Geometry: final body of the model. Coordinates: model frame, mm. A direction names the side the tool comes from. Coordinates: 2 decimals unless noted, no trailing zeros. Loops run counter-clockwise (first coordinate to the right, second up) from the corner with the lowest first, then second, coordinate; pieces in that order, holes last. Notation, with made-up numbers: (76.5, -35.5) - (111.5, -35.5) arc R13 cw to (111.5, -23.5) - close; hole circle Ø5 at (-18, 42). An arc over 180 degrees is marked (long way). Put each result on its own line as item: value. Start each with the question number.
1) Section A-A on z = 3. Output: boundary loops of the cut face in (x, y), and give its area (3 significant figures).
2) Section C-C on y = 42. Output: boundary loops of the cut face in (x, z).
3) Draft query along Z for faces 4 (the flat face through (33.6, 4, 1.6)), 5 (the cylindrical face through (-3.735, 2.028, 3.806)), 6 (the cylindrical face through (33.536, 2.028, 2.675)), 7 (the flat face through (15, 69, 0)). Return one class per face: +Z half, -Z half, draft (parallel to the pull), parting line (faces both ways), or undercut.
4) Section B-B on x = 35. Output: boundary loops of the cut face in (y, z), and give its area (3 significant figures).
5) Contact query for flat-ended pins moving along their axis: pin 1 Ø3 at (x, z) = (23.5, 4.5) entering from -Y; pin 2 Ø1 at (y, z) = (124.5, 3.5) entering from -X; pin 3 Ø1.8 at (x, z) = (-4, 3.5) entering from +Y; pin 4 Ø1.8 at (x, z) = (35, 3) entering from +Y. Output: stop coordinate, or through.
6) Material intervals for line 1 along X through (y, z) = (137, 1.35); line 2 along Y through (x, z) = (27, 3.5); line 3 along X through (y, z) = (1.25, 3), sorted ascending. Write a range as from..to.
7) Reachability of faces 1 (the flat face through (-6.4, 4, 1.6)), 2 (the flat face through (30, 71, 3)), 3 (the cylindrical face through (26.805, 138.487, 3.042)) from +Z, -Z, +X, -X, +Y, -Y: full face, straight path, thin tool, end or side. Return the list, or none.
```python
from build123d import *

# Parameters (mm, degrees)
SKETCH1_W           = 30
SKETCH1_H           = 140
BOSS_EXTRUDE1_DEPTH = 6
CHAMFER1_SIZE       = 2
SKETCH2_R           = 1.5
CUT_EXTRUDE1_DEPTH  = 6
SKETCH3_W           = 10
SKETCH3_H           = 6
BOSS_EXTRUDE2_DEPTH = 4
CHAMFER2_SIZE       = 2
SKETCH4_R           = 1.5
CUT_EXTRUDE2_DEPTH  = 142.887279204


with BuildPart() as part:
    # Sketch1 → Boss-Extrude1 (new body)
    with BuildSketch(Plane.XY):
        with Locations((15, 70)):
            Rectangle(SKETCH1_W, SKETCH1_H)
    extrude(amount=BOSS_EXTRUDE1_DEPTH)

    # Chamfer1
    chamfer1_edges = [part.edges().sort_by_distance(p)[0] for p in [
        (0, 140, 3),
        (30, 140, 3),
    ]]
    chamfer(chamfer1_edges, length=CHAMFER1_SIZE)

    # Sketch2 → Cut-Extrude1 (cut)
    with BuildSketch(Plane.XY.offset(6)):
        with Locations((3, 137)):
            Circle(SKETCH2_R)
        with Locations((27, 137)):
            Circle(SKETCH2_R)
    extrude(amount=-CUT_EXTRUDE1_DEPTH, mode=Mode.SUBTRACT)

    # Sketch3 → Boss-Extrude2 (add)
    with BuildSketch(Plane(origin=(0, 0, 0), x_dir=(1, 0, 0), z_dir=(0, 1, 0))):
        with Locations((-5, -3)):
            Rectangle(SKETCH3_W, SKETCH3_H)
        with Locations((35, -3)):
            Rectangle(SKETCH3_W, SKETCH3_H)
    extrude(amount=BOSS_EXTRUDE2_DEPTH)

    # Chamfer2
    chamfer2_edges = [part.edges().sort_by_distance(p)[0] for p in [
        (0, 4, 3),
        (-10, 4, 3),
        (30, 4, 3),
        (40, 4, 3),
    ]]
    chamfer(chamfer2_edges, length=CHAMFER2_SIZE)

    # Sketch4 → Cut-Extrude2 (cut, through all)
    with BuildSketch(Plane(origin=(0, 4, 0), x_dir=(1, 0, 0), z_dir=(0, 1, 0))):
        with Locations(Location((-5, -3, 0), (0, 0, 270))):
            Circle(SKETCH4_R)
        with Locations(Location((35, -3, 0), (0, 0, 270))):
            Circle(SKETCH4_R)
    extrude(amount=-CUT_EXTRUDE2_DEPTH, mode=Mode.SUBTRACT)


solid = part.part
```
Answer block:
1. outline: (-10, 0) - (-6.5, 0) - (-6.5, 4) - (-8, 4) - (-10, 2) - close; (-3.5, 0) - (33.5, 0) - (33.5, 4) - (32, 4) - (30, 6) - (30, 138) - (28, 140) - (2, 140) - (0, 138) - (0, 6) - (-2, 4) - (-3.5, 4) - close; (36.5, 0) - (40, 0) - (40, 2) - (38, 4) - (36.5, 4) - close; hole circle Ø3 at (3, 137); hole circle Ø3 at (27, 137)
1. area: 4,240 mm²
2. outline: (0, 0) - (30, 0) - (30, 6) - (0, 6) - close
3. face 4: draft
3. face 5: undercut
3. face 6: undercut
3. face 7: -Z half
4. outline: (0, 0) - (4, 0) - (4, 1.5) - (0, 1.5) - close; (0, 4.5) - (4, 4.5) - (4, 6) - (0, 6) - close
4. area: 12.0 mm²
5. pin 1: stops at y = 0
5. pin 2: stops at x = 0
5. pin 3: stops at y = 4
5. pin 4: passes through
6. line 1: x = 0..1.5, 4.5..25.5, 28.5..30
6. line 2: y = 0..135.5, 138.5..140
6. line 3: x = -10..-6.5, -3.5..33.5, 36.5..40
7. face 1: +Z, -Z, -X, +Y
7. face 2: +Z, -Z, +X, +Y
7. face 3: +Z, -Z
